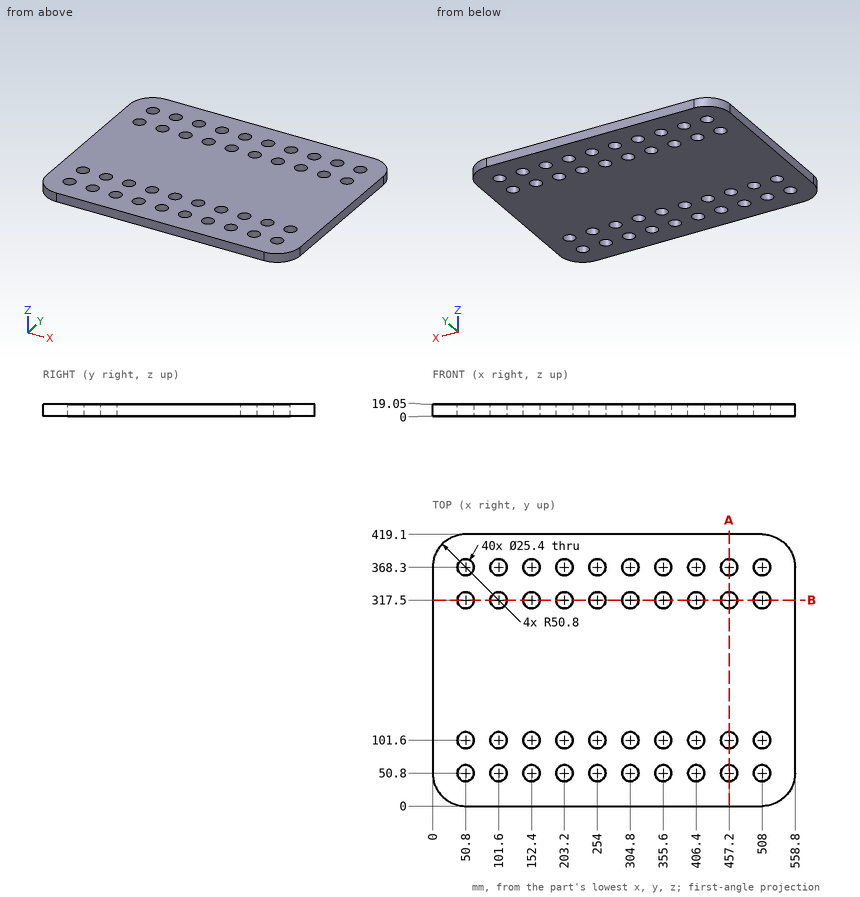
Input: dimensioned drawing with shaded views. Units: mm. Origin: part minimum x, y, z. Coordinates: 2 decimals unless noted, no trailing zeros. Order: outer loops, then holes, each group sorted by start corner. A loop starts at its lowest first (then second) coordinate and runs counter-clockwise, first axis right, second up.
1. Cut plane A-A, the plane x = 457.2. Return loops of the section in (y, z), plus the area to 3 significant figures.
Checked values:
outline: (0, 0) - (38.1, 0) - (38.1, 19.05) - (0, 19.05) - close; (63.5, 0) - (88.9, 0) - (88.9, 19.05) - (63.5, 19.05) - close; (114.3, 0) - (304.8, 0) - (304.8, 19.05) - (114.3, 19.05) - close; (330.2, 0) - (355.6, 0) - (355.6, 19.05) - (330.2, 19.05) - close; (381, 0) - (419.1, 0) - (419.1, 19.05) - (381, 19.05) - close
area: 6,050 mm2
2. Cut plane B-B, the plane y = 317.5. Count the separate pieces of the cut face and the enclosed holes in it, plus the area to 3 significant figures.
Checked values:
separate pieces: 11
enclosed holes: 0
area: 5,810 mm2
3. Ray query, line 1 along Y through (x, z) = (254, 5.5); line 2 along Y through (x, z) = (149, 1.5); line 3 along Y through (x, z) = (530, 14.75). Return the intervals inside material, ascending.
Checked values:
line 1: y = 0 to 38.1, 63.5 to 88.9, 114.3 to 304.8, 330.2 to 355.6, 381 to 419.1
line 2: y = 0 to 38.56, 63.04 to 89.36, 113.84 to 305.26, 329.74 to 356.06, 380.54 to 419.1
line 3: y = 5.01 to 414.09
